Source: three-view drawing plus pictorial views. Frame: mm from the lowest corner of the part. A direction names the side the tool comes from. Give positions to 0.01 mm unless a question says otherwise; leave off trailing zeros. Order: outer loops, then holes, each group sorted by start corner. A loop starts at its lowest first (then second) coordinate and runs counter-clockwise, first axis right, second up. Notation, with made-up numbers: (-33.75, -20.5) -> (0.25, -20.5) arc R19 cw to (0.25, 7.5) -> close; hole circle Ø6 at (11.5, -28). An arc over 180 degrees is marked (long way). Answer in a Markdown table with one row per item. Add a question column.
Q1. Pull-direction query (X, two-part tool) for the marked faces 1, 2, 3 and 4; classes: +X half, -X half, draft (parallel to the pull), parting line (faces both ways), or undercut.
Q2. Contact query for flat-ended pins moving along their axis: P1, Ø1.5, axis at x = 188, z = 27.5, coming from the +Y side; P2, Ø1.5, axis at x = 99, y = 26.5, coming from the -Z side; P3, Ø5, axis at x = 47, y = 32, coming from the -Z side. Output: stop coordinate, or through.
Q3. Cut plane C-C on y = 28.5. Return the cut outline in (x, z), and give its area (3 significant figures).
Q4. Set-up query: the marked faces 5 and 6. Return all of +Z, -Z, +X, -X, +Y, -Y with unobstructed straight access to the full face (end or side cutting, diameter ignored); none if empty.
Q5. Cut plane A-A on y = 15. Return the cut outline in (x, z), and give its area (3 significant figures).
Q6. Cut plane D-D on x = 78. Return the cut outline in (y, z).
Q7. Line query: line 1 along X through (y, z) = (7, 58.5); line 2 along X through (y, z) = (41, 18.5); line 3 along Y through (x, z) = (156.5, 12). Output: solid intervals per line, ascending. Write a range as from..to.
Q8. Cut plane B-B on z = 91.5. Return the cut outline in (x, y).
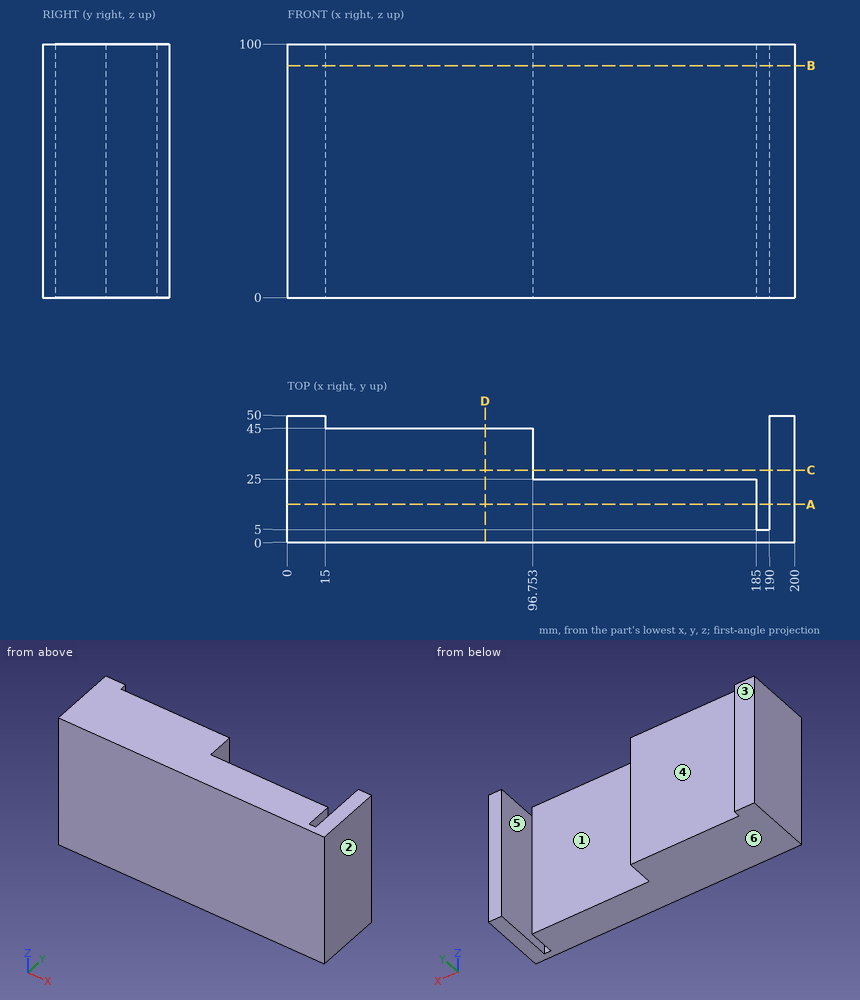
Completed:
| question | item | result |
|---|---|---|
| 1 | face 1 | undercut |
| 1 | face 2 | +X half |
| 1 | face 3 | draft |
| 1 | face 4 | undercut |
| 2 | P1 | stops at y = 5 |
| 2 | P2 | passes through |
| 2 | P3 | stops at z = 0 |
| 3 | outline | (0, 0) -> (96.75, 0) -> (96.75, 100) -> (0, 100) -> close; (190, 0) -> (200, 0) -> (200, 100) -> (190, 100) -> close |
| 3 | area | 10,700 mm² |
| 4 | face 5 | +Z, -Z, +Y |
| 4 | face 6 | -Z, +X, -X, +Y, -Y |
| 5 | outline | (0, 0) -> (185, 0) -> (185, 100) -> (0, 100) -> close; (190, 0) -> (200, 0) -> (200, 100) -> (190, 100) -> close |
| 5 | area | 19,500 mm² |
| 6 | outline | (0, 0) -> (45, 0) -> (45, 100) -> (0, 100) -> close |
| 7 | line 1 | x = 0..185, 190..200 |
| 7 | line 2 | x = 0..96.75, 190..200 |
| 7 | line 3 | y = 0..25 |
| 8 | outline | (0, 0) -> (200, 0) -> (200, 50) -> (190, 50) -> (190, 5) -> (185, 5) -> (185, 25) -> (96.75, 25) -> (96.75, 45) -> (15, 45) -> (15, 50) -> (0, 50) -> close |
